```python
from build123d import *

# Parameters (mm, degrees)
Y_KSEKLIK_EKSTR_ZYON1_DEPTH      = 230
Y_KSEKLIK_EKSTR_ZYON1_DEPTH_BACK = 230
IZIM1_R                          = 12.5
IZIM2_R                          = 4.25
KES_EKSTR_ZYON1_DEPTH            = 50
RADYUS1_R                        = 2


with BuildPart() as part:
    # izim1 → Y_kseklik-Ekstr_zyon1 (new, two sides: drawn at the far end of the back side and taken through both)
    with BuildSketch(Plane.XY.offset(-Y_KSEKLIK_EKSTR_ZYON1_DEPTH_BACK)):
        Circle(IZIM1_R)
    extrude(amount=Y_KSEKLIK_EKSTR_ZYON1_DEPTH + Y_KSEKLIK_EKSTR_ZYON1_DEPTH_BACK)

    # izim2 → Kes-Ekstr_zyon1 (cut)
    with BuildSketch(Plane(origin=(0, 0, 0), x_dir=(1, 0, 0), z_dir=(0, 1, 0))):
        with Locations(Location((0, 100, 0), (0, 0, 270))):
            Circle(IZIM2_R)
        with Locations(Location((0, -100, 0), (0, 0, 270))):
            Circle(IZIM2_R)
    extrude(amount=-KES_EKSTR_ZYON1_DEPTH, mode=Mode.SUBTRACT)

    # Radyus1
    radyus1_edges = [part.edges().sort_by_distance(p)[0] for p in [
        (-12.5, 0, 230),
        (-12.5, 0, -230),
    ]]
    fillet(radyus1_edges, radius=RADYUS1_R)


solid = part.part
```
Geometry: final body of the model. Coordinates: model frame, mm. A direction names the side the tool comes from. Round coordinates to 2 decimals unless told otherwise and drop trailing zeros. Loops run counter-clockwise (first coordinate to the right, second up) from the corner with the lowest first, then second, coordinate; pieces in that order, holes last. Notation, with made-up numbers: (-35.5, 77.25) -> (-4.5, 77.25) arc R14 cw to (-4.5, 87.25) -> close; hole circle Ø2 at (11, 26). An arc over 180 degrees is marked (long way). Use one line per item in the form item = value. Start each with the question number.
1) Section C-C on y = -4.5. Give the number of separate pieces and of enclosed holes in the cut face, then the cut area to 3 significant figures.
2) Section A-A on x = 0. Output: boundary loops of the cut face in (y, z).
3) Draft query along X for faces 3 (the flat face through (0, 0, -230)), 4 (the flat face through (0, 0, -100)), 5 (the cylindrical face through (-1.627, 12.394, -3.192)), 6 (the cylindrical face through (0.187, -6.166, 95.754)). Return one class per face: released by +X, released by -X, zero draft, split by the parting line, or undercut.
4) First-contact query: P1, Ø5, axis at x = 0, z = 100, coming from the -Y side; P2, Ø2, axis at y = -4, z = 99, coming from the -X side; P3, Ø10, axis at y = 5.5, z = -3, coming from the +X side. Flat tips, straight axial feed; report the tip coordinate or a pass-through.
5) Section B-B on z = 20. Output: boundary loops of the cut face in (x, y).
6) Section D-D on z = 100. Output: boundary loops of the cut face in (x, y).
7) Line query: L1, parallel to Z at x = 0, y = -9.5; L2, parallel to Z at x = -1.5, y = -9; L3, parallel to X at y = -4, z = 100. Output: solid intervals per line, ascending.
8) Access query for faces 1 (the flat face through (0, 0, 100)), 2 (the flat face through (0, 0, 230)). Directions: +Z, -Z, +X, -X, +Y, -Y. A direction counts if a zero-diameter tool reaches every point of the face in a straight line with its end or side. Return the directions, or none.
Response:
q1.separate_pieces = 1
q1.enclosed_holes = 2
q1.area = 10,600 mm^2
q2.outline = (-12.5, -228) arc R2 ccw to (-10.5, -230) -> (10.5, -230) arc R2 ccw to (12.5, -228) -> (12.5, 228) arc R2 ccw to (10.5, 230) -> (-10.5, 230) arc R2 ccw to (-12.5, 228) -> (-12.5, 104.25) -> (0, 104.25) -> (0, 95.75) -> (-12.5, 95.75) -> (-12.5, -95.75) -> (0, -95.75) -> (0, -104.25) -> (-12.5, -104.25) -> close
q3.face_3 = zero draft
q3.face_4 = undercut
q3.face_5 = split by the parting line
q3.face_6 = undercut
q4.P1 = 0
q4.P2 = -12.13
q4.P3 = 12.49
q5.outline = circle Ø25 at (0, 0)
q6.outline = (-4.25, -11.76) -> (-4.25, 0) -> (4.25, 0) -> (4.25, -11.76) arc R12.5 ccw (long way) to start
q7.L1 = -230 to -104.25, -95.75 to 95.75, 104.25 to 230
q7.L2 = -230 to -103.98, -96.02 to 96.02, 103.98 to 230
q7.L3 = -11.84 to -4.25, 4.25 to 11.84
q8.face_1 = -Y
q8.face_2 = +Z, +X, -X, +Y, -Y
